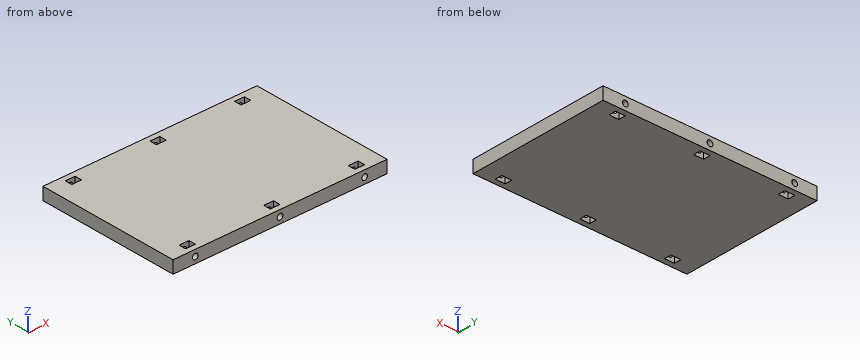
```python
from build123d import *

# Parameters (mm, degrees)
ESBO_O1_W                = 120
ESBO_O1_H                = 80
ESBO_O1_W_2              = 5.5
ESBO_O1_H_2              = 4
RESSALTO_EXTRUS_O4_DEPTH = 7
CORTE_EXTRUS_O1_START    = -80
ESBO_O2_R                = 1.6
CORTE_EXTRUS_O1_DEPTH    = 10
CORTE_EXTRUS_O2_START    = -10
ESBO_O2_2_R              = 1.6
CORTE_EXTRUS_O2_DEPTH    = 10


with BuildPart() as part:
    # Esboço1 → Ressalto-extrusão4 (new body)
    with BuildSketch(Plane.XY):
        Rectangle(ESBO_O1_W, ESBO_O1_H)
        with Locations((-47.46, -35)):
            Rectangle(ESBO_O1_W_2, ESBO_O1_H_2, mode=Mode.SUBTRACT)
        with Locations((47.46, -35)):
            Rectangle(ESBO_O1_W_2, ESBO_O1_H_2, mode=Mode.SUBTRACT)
        with Locations((0, -35)):
            Rectangle(ESBO_O1_W_2, ESBO_O1_H_2, mode=Mode.SUBTRACT)
        with Locations((47.46, 35)):
            Rectangle(ESBO_O1_W_2, ESBO_O1_H_2, mode=Mode.SUBTRACT)
        with Locations((0, 35)):
            Rectangle(ESBO_O1_W_2, ESBO_O1_H_2, mode=Mode.SUBTRACT)
        with Locations((-47.46, 35)):
            Rectangle(ESBO_O1_W_2, ESBO_O1_H_2, mode=Mode.SUBTRACT)
    extrude(amount=RESSALTO_EXTRUS_O4_DEPTH)

    # Esboço2 → Corte-extrusão1 (cut)
    with BuildSketch(Plane(origin=(0, 40, 0), x_dir=(1, 0, 0), z_dir=(0, 1, 0)).offset(CORTE_EXTRUS_O1_START)):
        with Locations(Location((-47.46, -3.5, 0), (0, 0, 270))):
            Circle(ESBO_O2_R)
        with Locations(Location((0, -3.5, 0), (0, 0, 270))):
            Circle(ESBO_O2_R)
        with Locations((47.46, -3.5)):
            Circle(ESBO_O2_R)
    extrude(amount=CORTE_EXTRUS_O1_DEPTH, mode=Mode.SUBTRACT)

    # Esboço2<2> → Corte-extrusão2 (cut)
    with BuildSketch(Plane(origin=(0, 40, 0), x_dir=(1, 0, 0), z_dir=(0, 1, 0)).offset(CORTE_EXTRUS_O2_START)):
        with Locations(Location((-47.46, -3.5, 0), (0, 0, 270))):
            Circle(ESBO_O2_2_R)
        with Locations(Location((0, -3.5, 0), (0, 0, 270))):
            Circle(ESBO_O2_2_R)
        with Locations((47.46, -3.5)):
            Circle(ESBO_O2_2_R)
    extrude(amount=CORTE_EXTRUS_O2_DEPTH, mode=Mode.SUBTRACT)


solid = part.part
```
Geometry check sheet. Reference: the model listing, model coordinates, mm. Coordinates: 2 decimals unless noted, no trailing zeros. Write each loop counter-clockwise with the first axis right and the second up, starting at its lowest first coordinate (ties: lowest second). Pieces come first, ordered by that corner, then holes. Notation, with made-up numbers: (30.25, 34) -> (54.25, 34) arc R13 cw to (54.25, 57) -> close; hole circle Ø10 at (31.5, 70). An arc over 180 degrees is marked (long way). Use CSV: the item, a comma, the result in double quotes. Start each with the question number.
Item 1: Cross-section at A-A, the plane x = 47.46. Record the cut outline in (y, z).
Item 2: Depth check by flat-ended pin: pin 1 Ø1 at (x, z) = (47.5, 3.5) entering from -Y; pin 2 Ø2.5 at (x, z) = (0, 3.5) entering from +Y. Enter the tip coordinate at first touch or a pass-through.
Item 3: Thickness scan on line 1 (Y direction, x = -46.5, z = 1.5); line 2 (X direction, y = 32.25, z = 3.5); line 3 (Z direction, x = 0, y = -31.5). Record the ranges inside material, lowest first.
Answers:
1,outline,"(-40, 0) -> (-37, 0) -> (-37, 1.9) -> (-40, 1.9) -> close; (-40, 5.1) -> (-37, 5.1) -> (-37, 7) -> (-40, 7) -> close; (-33, 0) -> (33, 0) -> (33, 1.9) -> (30, 1.9) -> (30, 5.1) -> (33, 5.1) -> (33, 7) -> (-33, 7) -> (-33, 5.1) -> (-30, 5.1) -> (-30, 1.9) -> (-33, 1.9) -> close; (37, 0) -> (40, 0) -> (40, 1.9) -> (37, 1.9) -> close; (37, 5.1) -> (40, 5.1) -> (40, 7) -> (37, 7) -> close"
2,pin 1,"y = -30"
2,pin 2,"y = 30"
3,line 1,"-40 to -37, -33 to 33, 37 to 40"
3,line 2,"-60 to -49.06, -45.86 to -1.6, 1.6 to 45.86, 49.06 to 60"
3,line 3,"0 to 1.9, 5.1 to 7"
